Part model, mm, in its own coordinate system. A direction names the side the tool comes from. Give positions to 0.01 mm unless a question says otherwise; leave off trailing zeros. Write each loop counter-clockwise with the first axis right and the second up, starting at its lowest first coordinate (ties: lowest second). Pieces come first, ordered by that corner, then holes. Notation, with made-up numbers: M 1.25,85 L 45.25,85 A25 ccw 45.25,114 Z; hole C 43.25,87 d8. An arc over 180 degrees is marked long. Answer as CSV lines item,"result". Start each with the question number.
Item 1: Band-saw the part on D-D, the plane x = -3. List the corners of the cut face in (y, z) (3 decimals).
Item 2: Band-saw the part on C-C, the plane z = -21. List the corners of the cut face in (x, y) (3 decimals), then the cut area to 3 significant figures.
Item 3: 3-axis set-ups, long thin cutter, end or side, ignore diameter. For faces 1 (the flat face through (20, -6.35, 91)), 2 (the flat face through (15.875, -33, 12)), 3 (the flat face through (0.13, 18.05, 63.18)): which of +Z, -Z, +X, -X, +Y, -Y reach the whole face in a straight line?
Item 4: Wall check: L1, parallel to Y at x = -6, z = 0 (3 decimals); L2, parallel to Z at x = 45, y = -27.5 (3 decimals); L3, parallel to Y at x = 31.75, z = 95.25 (3 decimals). Give the ranges that are in metal, low to high. Write a range as from..to.
Item 5: Two-plate mould, pull along Z, no slides. Class faces 4 (the flat face through (-9.525, -24, 63)), 5 (the flat face through (15, -29, 101.6)), 6 (the flat face through (22, -19, 79.375)): +Z half, -Z half, draft (parallel to the pull), parting line (faces both ways), or undercut.
Item 6: Band-saw the part on A-A, the plane x = 25. List the corners of the cut face in (y, z) (3 decimals).
Item 7: Band-saw the part on B-B, the plane y = 19. List the corners of the cut face in (x, z) (3 decimals).
Item 8: Pin check, flat tips, straight feed: pin 1 (10 mm diameter, centred on x = 26, y = -32.5, fed in from -Z); pin 2 (3 mm diameter, centred on y = 38.5, z = 10.5, fed in from +X) (3 decimals); pin 3 (2 mm diameter, centred on x = -2, y = 32.5, fed in from -Z); pin 4 (3 mm diameter, centred on x = -4.5, y = 40, fed in from -Z). Stop position of each tip, or through.
from build123d import *

# Parameters (mm, degrees)
SKETCH1_R           = 50.8
SKETCH1_R_2         = 34.925
BOSS_EXTRUDE1_DEPTH = 9.525
SKETCH1_3_R         = 50.8
SKETCH1_3_R_2       = 34.925
BOSS_EXTRUDE2_DEPTH = 15.875
SKETCH2_W           = 22.225
SKETCH2_H           = 44.45
BOSS_EXTRUDE3_DEPTH = 50.8
SKETCH3_R           = 12.7
CUT_EXTRUDE1_DEPTH  = 153.4


with BuildPart() as part:
    # Sketch1 → Boss-Extrude1 (new body, symmetric)
    with BuildSketch(Plane(origin=(0, 0, 0), x_dir=(0, 0, -1), z_dir=(1, 0, 0))):
        Circle(SKETCH1_R)
        Circle(SKETCH1_R_2, mode=Mode.SUBTRACT)
        with BuildLine():
            Line((-101.6, -50.8), (0, -50.8))
            ThreePointArc((0, -50.8), (-48.489607735, -15.145888606), (-28.914102256, 41.768584974))
            Line((-28.914102256, 41.768584974), (-98.425, -6.35))
            Line((-98.425, -6.35), (-101.6, -6.35))
            Line((-101.6, -6.35), (-101.6, -50.8))
        make_face()
    extrude(amount=BOSS_EXTRUDE1_DEPTH, both=True)

    # Sketch1_3 → Boss-Extrude2 (add, symmetric)
    with BuildSketch(Plane(origin=(0, 0, 0), x_dir=(0, 0, -1), z_dir=(1, 0, 0))):
        Circle(SKETCH1_3_R)
        Circle(SKETCH1_3_R_2, mode=Mode.SUBTRACT)
    extrude(amount=BOSS_EXTRUDE2_DEPTH, both=True)

    # Sketch2 → Boss-Extrude3 (add)
    with BuildSketch(Plane(origin=(9.525, 0, 0), x_dir=(0, 0, -1), z_dir=(1, 0, 0))):
        with Locations((-90.4875, -28.575)):
            Rectangle(SKETCH2_W, SKETCH2_H)
    extrude(amount=BOSS_EXTRUDE3_DEPTH)

    # Sketch3 → Cut-Extrude1 (cut, through all)
    with BuildSketch(Plane.XY.offset(101.6)):
        with BuildLine():
            Line((60.325, -6.35), (31.75, -6.35))
            ThreePointArc((31.75, -6.35), (53.975, -28.575), (31.75, -50.8))
            Line((31.75, -50.8), (60.325, -50.8))
            Line((60.325, -50.8), (60.325, -6.35))
        make_face()
        with Locations((31.75, -28.575)):
            Circle(SKETCH3_R)
    extrude(amount=-CUT_EXTRUDE1_DEPTH, mode=Mode.SUBTRACT)


solid = part.part
Output:
1,outline,"M -50.8,0 A50.8 ccw long 41.769,28.914 L -6.35,98.425 L -6.35,101.6 L -50.8,101.6 Z; hole C 0,0 d69.85"
2,outline,"M -15.875,-46.256 L 15.875,-46.256 L 15.875,-27.906 L -15.875,-27.906 Z; M -15.875,27.906 L 15.875,27.906 L 15.875,46.256 L -15.875,46.256 Z"
2,area,"1,170 mm²"
3,face 1,"+Z, +X, +Y"
3,face 2,"-Z, +X, +Y, -Y"
3,face 3,"+Z, +X, -X, +Y"
4,L1,"-50.8..-34.925, 34.925..50.8"
4,L2,"79.375..101.6"
4,L3,"-50.8..-41.275, -15.875..-6.35"
5,face 4,"draft"
5,face 5,"+Z half"
5,face 6,"undercut"
6,outline,"M -50.8,79.375 L -39.333,79.375 L -39.333,101.6 L -50.8,101.6 Z; M -17.817,79.375 L -6.35,79.375 L -6.35,101.6 L -17.817,101.6 Z"
7,outline,"M -15.875,-47.113 L 15.875,-47.113 L 15.875,-29.305 L -15.875,-29.305 Z; M -15.875,29.305 L 15.875,29.305 L 15.875,47.113 L 9.525,47.113 L 9.525,61.805 L -9.525,61.805 L -9.525,47.113 L -15.875,47.113 Z"
8,pin 1,"through"
8,pin 2,"x = 15.875"
8,pin 3,"z = -39.85"
8,pin 4,"z = -33.14"
